Verification items for the finished model (mm, model axes). Give positions to 0.01 mm unless a question says otherwise; leave off trailing zeros. Write each loop counter-clockwise with the first axis right and the second up, starting at its lowest first coordinate (ties: lowest second). Pieces come first, ordered by that corner, then holes. Notation, with made-up numbers: M -40,52.25 L -16,52.25 A20 ccw -16,64.25 Z; hole C 24,-9 d11. An arc over 180 degrees is marked long. Answer as a JSON object with one key per item and string values.
```python
from build123d import *

# Parameters (mm, degrees)
F0_W     = 88.9
F0_H     = 152.4
F1_DEPTH = 5.08
F3_DEPTH = 25.4
F4_R     = 1.5875
F5_DEPTH = 25.4
F6_R     = 5.08


with BuildPart() as f1:
    # F0 (on Top) → F1 (new body)
    with BuildSketch(Plane.XY):
        with Locations((44.45, -76.2)):
            Rectangle(F0_W, F0_H)
    extrude(amount=F1_DEPTH)

    # F2 (on face) → F3 (cut)
    with BuildSketch(Plane.XY.offset(5.08)):
        Polygon((78.105, 0), (10.795, 0), (10.795, -10.16), (18.415, -15.24), (18.415, -35.56), (10.795, -50.8), (10.795, -129.54), (78.105, -129.54), (78.105, -50.8), (70.485, -35.56), (70.485, -15.24), (78.105, -10.16), align=None)
    extrude(amount=-F3_DEPTH, mode=Mode.SUBTRACT)

    # F4 (on face) → F5 (cut)
    with BuildSketch(Plane.XY.offset(5.08)):
        with Locations((5.08, -5.08)):
            Circle(F4_R)
        with Locations((83.82, -5.08)):
            Circle(F4_R)
        with Locations((83.82, -147.32)):
            Circle(F4_R)
        with Locations((5.08, -147.32)):
            Circle(F4_R)
    extrude(amount=-F5_DEPTH, mode=Mode.SUBTRACT)

    # F6
    f6_edges = [f1.edges().sort_by_distance(p)[0] for p in [
        (88.9, -152.4, 2.54),
        (0, -152.4, 2.54),
        (88.9, 0, 2.54),
        (0, 0, 2.54),
        (18.415, -15.24, 2.54),
        (18.415, -35.56, 2.54),
        (70.485, -35.56, 2.54),
        (70.485, -15.24, 2.54),
    ]]
    fillet(f6_edges, radius=F6_R)


solid = f1.part
```
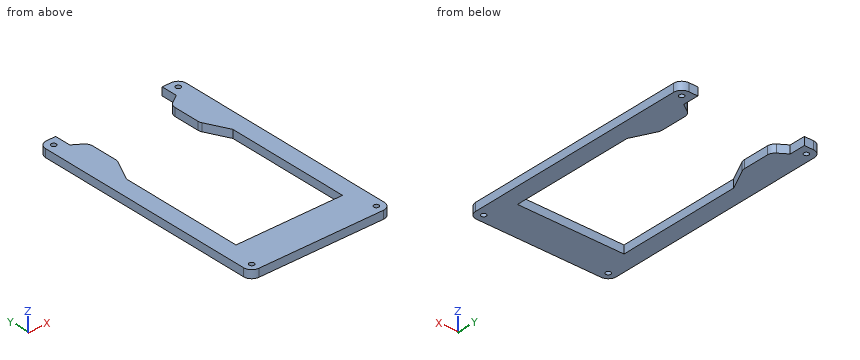
1) Section check B-B on z = 3.1. Record the boundary of the cut face in (x, y) (1 decimal), and give its area (3 significant figures).
Completed:
{"outline": "M 0,-147.3 A5.1 ccw 5.1,-152.4 L 83.8,-152.4 A5.1 ccw 88.9,-147.3 L 88.9,-5.1 A5.1 ccw 83.8,0 L 78.1,0 L 78.1,-10.2 L 72.7,-13.7 A5.1 ccw 70.5,-18 L 70.5,-34.4 A5.1 ccw 71,-36.6 L 78.1,-50.8 L 78.1,-129.5 L 10.8,-129.5 L 10.8,-50.8 L 17.9,-36.6 A5.1 ccw 18.4,-34.4 L 18.4,-18 A5.1 ccw 16.2,-13.7 L 10.8,-10.2 L 10.8,0 L 5.1,0 A5.1 ccw 0,-5.1 Z; hole C 5.1,-147.3 d3.2; hole C 5.1,-5.1 d3.2; hole C 83.8,-147.3 d3.2; hole C 83.8,-5.1 d3.2", "area": "5,240 mm2"}
2) Section check D-D on x = 51.5. Record the boundary of the cut face in (y, z), and give its area (3 significant figures).
Completed:
{"outline": "M -152.4,0 L -129.54,0 L -129.54,5.08 L -152.4,5.08 Z", "area": "116 mm2"}
3) Section check C-C on y = -30. Record the boundary of the cut face in (x, z) (3 decimals), and give its area (3 significant figures).
Completed:
{"outline": "M 0,0 L 18.415,0 L 18.415,5.08 L 0,5.08 Z; M 70.485,0 L 88.9,0 L 88.9,5.08 L 70.485,5.08 Z", "area": "187 mm2"}
4) Go/stop test with flat-tipped pins: pin 1 (1.9 mm diameter, centred on x = 5.08, y = -5.08, fed in from -Z); pin 2 (2.5 mm diameter, centred on x = 61, z = 3.5, fed in from +Y). Record where each tip stops, or that it passes through.
Completed:
{"pin 1": "passes through", "pin 2": "stops at y = -129.54"}
5) Thickness scan on L1, parallel to Y at x = 83.5, z = 1.45; L2, parallel to Y at x = 5.08, z = 2.35; L3, parallel to X at y = -65, z = 2.5 (3 decimals). Record the ranges inside material, lowest first.
Completed:
{"L1": "y = -152.4 to -148.87, -145.77 to -6.63, -3.53 to 0", "L2": "y = -152.4 to -148.91, -145.73 to -6.67, -3.49 to 0", "L3": "x = 0 to 10.795, 78.105 to 88.9"}
6) Section check A-A on y = -94. Record the boundary of the cut face in (x, z) (3 decimals), and give its area (3 significant figures).
Completed:
{"outline": "M 0,0 L 10.795,0 L 10.795,5.08 L 0,5.08 Z; M 78.105,0 L 88.9,0 L 88.9,5.08 L 78.105,5.08 Z", "area": "110 mm2"}
